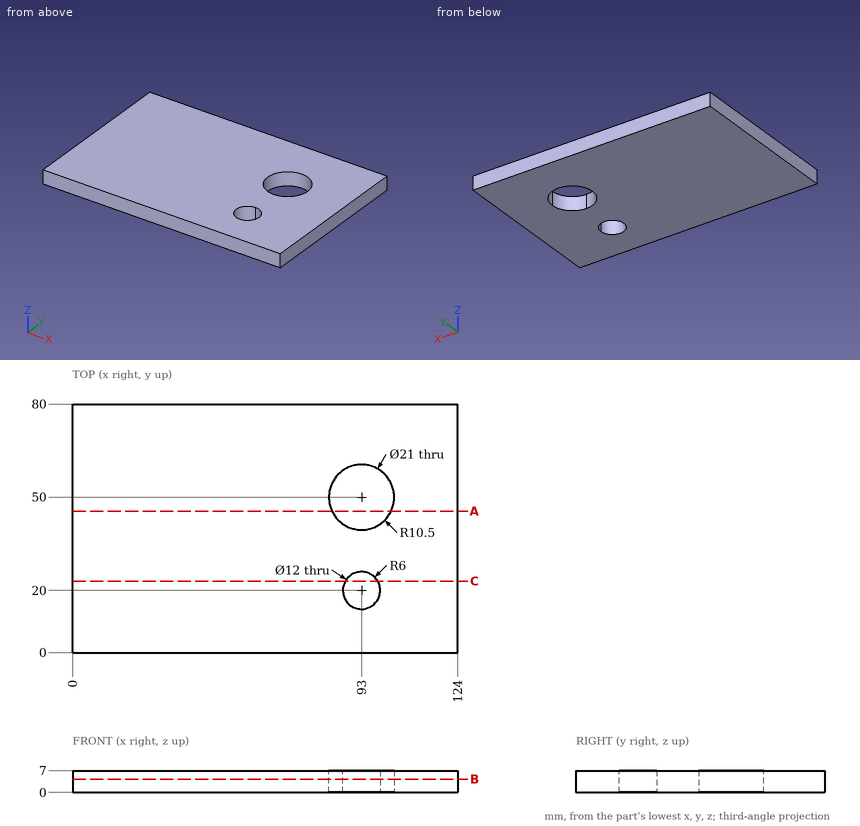
Answer from the drawing. Dimensions are ordinates in mm from the lowest x, y and z of the part. Give positions to 0.01 mm unless a question says otherwise; leave off trailing zeros. Loops run counter-clockwise (first coordinate to the right, second up) from the corner with the lowest first, then second, coordinate; pieces in that order, holes last. Notation, with made-up numbers: (52.25, 24) -> (104.25, 24) arc R13 cw to (104.25, 45) -> close; hole circle Ø10 at (46.25, 74). An arc over 180 degrees is marked (long way). Use a Markdown table: item, result.
Q1. Section B-B, the plane z = 4.25 is taken. Determine the outline of the cut face in (x, y).
Solved:
| item | result |
|---|---|
| outline | (0, 0) -> (124, 0) -> (124, 80) -> (0, 80) -> close; hole circle Ø21 at (93, 50); hole (93, 26) arc R6 ccw (long way) to (99, 20) arc R6 ccw to start |
Q2. Section A-A, the plane y = 45.5 is taken. Determine the outline of the cut face in (x, z), then the cut area to 3 significant figures.
Solved:
| item | result |
|---|---|
| outline | (0, 0) -> (83.51, 0) -> (83.51, 7) -> (0, 7) -> close; (102.49, 0) -> (124, 0) -> (124, 7) -> (102.49, 7) -> close |
| area | 735 mm^2 |
Q3. This flat-tipped pin is pushed along its axis until it touches: pin 1 (12.5 mm diameter, centred on x = 93, y = 50, fed in from +Z). Where does it stop, or does it pass through?
Solved:
| item | result |
|---|---|
| pin 1 | passes through |
Q4. Section C-C, the plane y = 23 is taken. Determine the outline of the cut face in (x, z), then the cut area to 3 significant figures.
Solved:
| item | result |
|---|---|
| outline | (0, 0) -> (87.8, 0) -> (87.8, 7) -> (0, 7) -> close; (98.2, 0) -> (124, 0) -> (124, 7) -> (98.2, 7) -> close |
| area | 795 mm^2 |
Q5. Find the intervals of material crossed by line 1 along Y through (x, z) = (93, 1.5); line 2 along X through (y, z) = (50, 4); line 3 along X through (y, z) = (20, 1.75), in increasing order.
Solved:
| item | result |
|---|---|
| line 1 | y = 0 to 14, 26 to 39.5, 60.5 to 80 |
| line 2 | x = 0 to 82.5, 103.5 to 124 |
| line 3 | x = 0 to 87, 99 to 124 |
